```python
from build123d import *

# Parameters (mm, degrees)
F1_DEPTH = 38.1
F2_R     = 12.7
F3_DEPTH = 50.9263650248
F4_ANGLE = 90
F5_R     = 12.7


with BuildPart() as f1:
    # F0 (on Top) → F1 (new body)
    with BuildSketch(Plane.XY):
        with BuildLine():
            ThreePointArc((0, 15.875), (11.2253201513, 11.2253201513), (15.875, 0))
            ThreePointArc((15.875, 0), (11.2253201513, -11.2253201513), (0, -15.875))
            Line((0, -15.875), (0, -25.5253650248))
            Line((0, -25.5253650248), (76.2, -25.5253650248))
            Line((76.2, -25.5253650248), (76.2, 25.4))
            Line((76.2, 25.4), (0, 25.4))
            Line((0, 25.4), (0, 15.875))
        make_face()
        with BuildLine():
            ThreePointArc((0, -15.875), (-15.875, 0), (0, 15.875))
            Line((0, 15.875), (0, 25.4))
            Line((0, 25.4), (-76.2, 25.4))
            Line((-76.2, 25.4), (-76.2, -25.5253650248))
            Line((-76.2, -25.5253650248), (0, -25.5253650248))
            Line((0, -25.5253650248), (0, -15.875))
        make_face()
    extrude(amount=F1_DEPTH)

    # F2 (on face) → F3 (cut, through all)
    with BuildSketch(Plane(origin=(0, 25.4, 0), x_dir=(-1, 0, 0), z_dir=(0, 1, 0))):
        with Locations((-38.1, 19.05)):
            Circle(F2_R)
        with Locations((38.1, 19.05)):
            Circle(F2_R)
    extrude(amount=-F3_DEPTH, mode=Mode.SUBTRACT)


with BuildPart() as f1_1:
    # F4: moved
    add(f1.part.rotate(Axis((0, -25.5253650248, 38.1), (1, 0, 0)), F4_ANGLE))

    # F5
    f5_edges = [f1_1.edges().sort_by_distance(p)[0] for p in [
        (76.2, -25.525365, 63.562683),
        (76.2, 12.574635, 63.562683),
        (-76.2, -25.525365, 63.562683),
        (-76.2, 12.574635, 63.562683),
    ]]
    fillet(f5_edges, radius=F5_R)


with BuildPart() as f6_1:
    # F6: copy of F1
    add(f1_1.part.moved(Location((0, 0, 70.31364))))


solid = f1_1.part
```
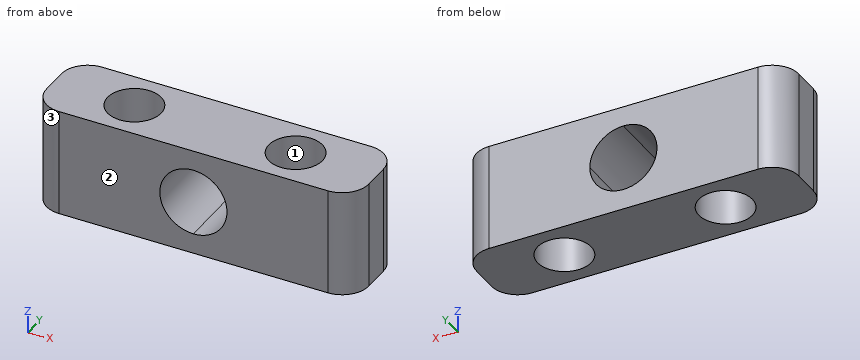
Source: CAD feature listing. Evaluate the final solid. Frame: model axes, mm. Face numbers are marked on the shaded views. Coordinates: 2 decimals unless noted, no trailing zeros. Loops run counter-clockwise (first coordinate to the right, second up) from the corner with the lowest first, then second, coordinate; pieces in that order, holes last. Notation, with made-up numbers: M 31,-7.75 L 51,-7.75 A11 ccw 51,-2.75 Z; hole C -13.75,88 d11. An arc over 180 degrees is marked long. Use a Markdown table: item, result. Add a question column.
Q1. Draft query along X for the marked faces 1, 2 and 3. Return one class per face: pulls with the +X half, pulls with the -X half, needs draft (parallel to the pull), parting line crosses it, or undercut.
Q2. Section query A-A, the plane z = 62. Return loops of the section in (x, y).
Q3. Material intervals for L1, parallel to Y at x = -38, z = 78; L2, parallel to X at y = -4.5, z = 62.5; L3, parallel to X at y = -17.5, z = 84, sorted ascending.
Q4. Section query B-B, the plane x = -38.1. Return loops of the section in (y, z), and give its area (3 significant figures).
Q5. Section query C-C, the plane y = -21. Return loops of the section in (x, z) (3 decimals).
Q6. Section query D-D, the plane z = 56. Return loops of the section in (x, y), and give its area (3 significant figures).
Result:
| question | item | result |
|---|---|---|
| 1 | face 1 | undercut |
| 1 | face 2 | needs draft |
| 1 | face 3 | pulls with the -X half |
| 2 | outline | M -76.2,-12.83 A12.7 ccw -63.5,-25.53 L -15.79,-25.53 L -15.79,12.57 L -63.5,12.57 A12.7 ccw -76.2,-0.13 Z; M 15.79,-25.53 L 63.5,-25.53 A12.7 ccw 76.2,-12.83 L 76.2,-0.13 A12.7 ccw 63.5,12.57 L 15.79,12.57 Z; hole C -38.1,-6.48 d25.4; hole C 38.1,-6.48 d25.4 |
| 3 | L1 | y = -25.53 to -19.17, 6.22 to 12.57 |
| 3 | L2 | x = -76.2 to -50.65, -25.55 to -15.84, 15.84 to 25.55, 50.65 to 76.2 |
| 3 | L3 | x = -75.31 to -44.4, -31.8 to 31.8, 44.4 to 75.31 |
| 4 | outline | M -25.53,38.1 L -19.18,38.1 L -19.18,89.03 L -25.53,89.03 Z; M 6.22,38.1 L 12.57,38.1 L 12.57,89.03 L 6.22,89.03 Z |
| 4 | area | 647 mm2 |
| 5 | outline | M -73.219,38.1 L 73.219,38.1 L 73.219,89.025 L -73.219,89.025 Z; hole C 0,63.625 d31.75 |
| 6 | outline | M -76.2,-12.83 A12.7 ccw -63.5,-25.53 L -13.92,-25.53 L -13.92,12.57 L -63.5,12.57 A12.7 ccw -76.2,-0.13 Z; M 13.92,-25.53 L 63.5,-25.53 A12.7 ccw 76.2,-12.83 L 76.2,-0.13 A12.7 ccw 63.5,12.57 L 13.92,12.57 Z; hole C -38.1,-6.48 d25.4; hole C 38.1,-6.48 d25.4 |
| 6 | area | 3,590 mm2 |
